Can you work these out from the model? Positions are in its coordinate system, mm. Face numbers are marked on the shaded views. A direction names the side the tool comes from. Round coordinates to 2 decimals unless told otherwise and drop trailing zeros. Write each loop counter-clockwise with the first axis right and the second up, starting at its lowest first coordinate (ties: lowest second). Pieces come first, ordered by that corner, then holes. Notation, with made-up numbers: M 18,54 L 61,54 A11 cw 61,66 Z; hole C 80,27 d5. An arc over 180 degrees is marked long. Answer in a Markdown table with one row per item. Add a question column.
(1) Suppose I cut it at C-C, the plane y = -4.7. Write out the boundary of the cut face in (x, z), then the cut area to 3 significant figures.
(2) I'm going to push flat-ended pins straight in: pin 1 (9 mm diameter, centred on x = 0.5, z = -14, fed in from -Y); pin 2 (0.9 mm diameter, centred on x = -1.5, y = -4.5, fed in from +Z); pin 3 (3 mm diameter, centred on x = -1.5, z = -0.5, fed in from -Y). Where does each tip first touch, or does it pass through?
(3) Suppose I cut it at A-A, the plane z = 0.5. Write out the boundary of the cut face in (x, y), then the cut area to 3 significant figures.
(4) If I drill on probe 1 along X at (y, z) = (-4.2, 11); probe 2 along Y at (x, z) = (-7.75, 8); probe 3 along Z at (x, y) = (-1.5, -5.3), over which ranges is the centre line in solid material (lowest first)?
(5) For the marked faces 4, 5 and 6, which set-ups out of +Z, -Z, +X, -X, +Y, -Y let a thin tool reach every point of the face, with its end or its side?
(6) If we mould it in two halves opening along X, with no side actions, what happens to the marked faces 1, 2 and 3? For each: released by +X, released by -X, zero draft, split by the parting line, or undercut.
(7) Suppose I cut it at B-B, the plane x = -1.25. Write out the boundary of the cut face in (y, z).
from build123d import *

# Parameters (mm, degrees)
F0_W     = 23
F0_H     = 60
F1_DEPTH = 6
F2_T     = -2.5
F3_W     = 23
F3_H     = 6
F4_DEPTH = 7
F5_W     = 23
F5_H     = 6
F6_DEPTH = 7
F7_W     = 18
F7_H     = 4
F8_DEPTH = 3


with BuildPart() as f1:
    # F0 (on Front) → F1 (new body)
    with BuildSketch(Plane.XZ):
        Rectangle(F0_W, F0_H)
    extrude(amount=F1_DEPTH)

    # F2
    f2_openings = [f1.faces().sort_by_distance(p)[0] for p in [
        (0, -6, 0),
    ]]
    offset(amount=F2_T, openings=f2_openings)

    # F3 (on face) → F4 (cut)
    with BuildSketch(Plane(origin=(0, 0, -30), x_dir=(1, 0, 0), z_dir=(0, 0, -1))):
        with Locations((0, 3)):
            Rectangle(F3_W, F3_H)
    extrude(amount=-F4_DEPTH, mode=Mode.SUBTRACT)

    # F5 (on face) → F6 (cut)
    with BuildSketch(Plane.XY.offset(30)):
        with Locations((0, -3)):
            Rectangle(F5_W, F5_H)
    extrude(amount=-F6_DEPTH, mode=Mode.SUBTRACT)

    # F7 (on face) → F8 (join)
    with BuildSketch(Plane.XZ.offset(2.5)):
        Rectangle(F7_W, F7_H)
    extrude(amount=F8_DEPTH)


solid = f1.part
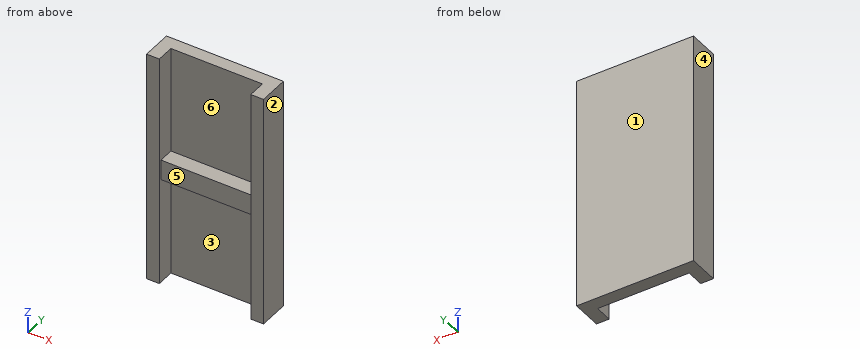
Calculated:
| question | item | result |
|---|---|---|
| 1 | outline | M -11.5,-23 L -9,-23 L -9,-2 L 9,-2 L 9,-23 L 11.5,-23 L 11.5,23 L 9,23 L 9,2 L -9,2 L -9,23 L -11.5,23 Z |
| 1 | area | 302 mm² |
| 2 | pin 1 | y = -2.5 |
| 2 | pin 2 | z = 2 |
| 2 | pin 3 | y = -5.5 |
| 3 | outline | M -11.5,-6 L -9,-6 L -9,-5.5 L 9,-5.5 L 9,-6 L 11.5,-6 L 11.5,0 L -11.5,0 Z |
| 3 | area | 129 mm² |
| 4 | probe 1 | -11.5 to -9, 9 to 11.5 |
| 4 | probe 2 | -2.5 to 0 |
| 4 | probe 3 | -2 to 2 |
| 5 | face 4 | +Z, -Z, -X, +Y, -Y |
| 5 | face 5 | +Z, -Z, -Y |
| 5 | face 6 | +Z, -Y |
| 6 | face 1 | zero draft |
| 6 | face 2 | released by +X |
| 6 | face 3 | undercut |
| 7 | outline | M -5.5,-2 L -2.5,-2 L -2.5,-23 L 0,-23 L 0,23 L -2.5,23 L -2.5,2 L -5.5,2 Z |
